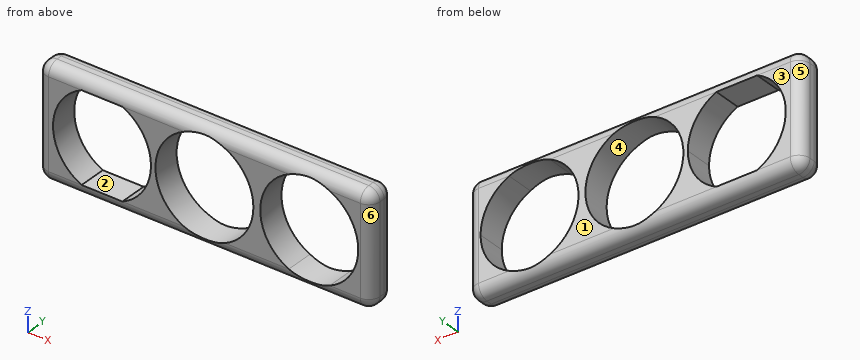
from build123d import *

# Parameters (mm, degrees)
F0_W         = 76.2
F0_H         = 25.4
F0_R         = 11.176
F1_DEPTH     = 6.35
F2_T1_DEPTH  = 71.12
F2_T3_DEPTH  = 1.27
F2_T5_DEPTH  = 20.32
F2_S9_W      = 2.54
F2_S9_H      = 2.54
F2_T10_DEPTH = 2.54
F2_S15_W     = 2.54
F2_S15_H     = 2.54
F2_T16_DEPTH = 2.54
F2_S21_W     = 2.54
F2_S21_H     = 2.54
F2_T22_DEPTH = 2.54
F2_S27_W     = 2.54
F2_S27_H     = 2.54
F2_T28_DEPTH = 2.54
F2_S33_W     = 2.54
F2_S33_H     = 2.54
F2_T34_DEPTH = 2.54
F2_S39_W     = 2.54
F2_S39_H     = 2.54
F2_T40_DEPTH = 2.54
F2_S45_W     = 2.54
F2_S45_H     = 2.54
F2_T46_DEPTH = 2.54
F2_S51_W     = 2.54
F2_S51_H     = 2.54
F2_T52_DEPTH = 2.54
F4_DEPTH     = 6.35


# Not quite as in the source:
# - a fillet or chamfer that OpenCascade refuses, or shapes differently, is made with other operations: its cross-section is extruded or revolved along the edge and cut away or added


with BuildPart() as f1:
    # F0 (on Front) → F1 (new body)
    with BuildSketch(Plane.XZ):
        Rectangle(F0_W, F0_H)
        Circle(F0_R, mode=Mode.SUBTRACT)
    extrude(amount=F1_DEPTH)

    # F2: fillet of radius 2.54 on 12 edges, made by hand

    # F2_s2 → F2_t1 (cut)
    with BuildSketch(Plane.YZ.offset(-35.56)):
        with BuildLine():
            ThreePointArc((-2.54, -12.7), (-0.7439487758, -11.9560512242), (0, -10.16))
            Line((0, -10.16), (0, -12.7))
            Line((0, -12.7), (-2.54, -12.7))
        make_face()
        with BuildLine():
            ThreePointArc((-3.81, -12.7), (-5.6060512242, -11.9560512242), (-6.35, -10.16))
            Line((-6.35, -10.16), (-6.35, -12.7))
            Line((-6.35, -12.7), (-3.81, -12.7))
        make_face()
        with BuildLine():
            ThreePointArc((-2.54, 12.7), (-0.7439487758, 11.9560512242), (0, 10.16))
            Line((0, 10.16), (0, 12.7))
            Line((0, 12.7), (-2.54, 12.7))
        make_face()
        with BuildLine():
            ThreePointArc((-3.81, 12.7), (-5.6060512242, 11.9560512242), (-6.35, 10.16))
            Line((-6.35, 10.16), (-6.35, 12.7))
            Line((-6.35, 12.7), (-3.81, 12.7))
        make_face()
    extrude(amount=F2_T1_DEPTH, mode=Mode.SUBTRACT)

    # F2_s4 → F2_t3 (cut)
    with BuildSketch(Plane.XZ.offset(2.54)):
        with BuildLine():
            ThreePointArc((-38.1, -10.16), (-37.3560512242, -11.9560512242), (-35.56, -12.7))
            Line((-35.56, -12.7), (-38.1, -12.7))
            Line((-38.1, -12.7), (-38.1, -10.16))
        make_face()
        with BuildLine():
            ThreePointArc((38.1, -10.16), (37.3560512242, -11.9560512242), (35.56, -12.7))
            Line((35.56, -12.7), (38.1, -12.7))
            Line((38.1, -12.7), (38.1, -10.16))
        make_face()
        with BuildLine():
            ThreePointArc((38.1, 10.16), (37.3560512242, 11.9560512242), (35.56, 12.7))
            Line((35.56, 12.7), (38.1, 12.7))
            Line((38.1, 12.7), (38.1, 10.16))
        make_face()
        with BuildLine():
            ThreePointArc((-35.56, 12.7), (-37.3560512242, 11.9560512242), (-38.1, 10.16))
            Line((-38.1, 10.16), (-38.1, 12.7))
            Line((-38.1, 12.7), (-35.56, 12.7))
        make_face()
    extrude(amount=F2_T3_DEPTH, mode=Mode.SUBTRACT)

    # F2_s6 → F2_t5 (cut)
    with BuildSketch(Plane.XY.offset(-10.16)):
        with BuildLine():
            ThreePointArc((-38.1, -3.81), (-37.3560512242, -5.6060512242), (-35.56, -6.35))
            Line((-35.56, -6.35), (-38.1, -6.35))
            Line((-38.1, -6.35), (-38.1, -3.81))
        make_face()
        with BuildLine():
            ThreePointArc((-38.1, -2.54), (-37.3560512242, -0.7439487758), (-35.56, 0))
            Line((-35.56, 0), (-38.1, 0))
            Line((-38.1, 0), (-38.1, -2.54))
        make_face()
        with BuildLine():
            ThreePointArc((38.1, -3.81), (37.3560512242, -5.6060512242), (35.56, -6.35))
            Line((35.56, -6.35), (38.1, -6.35))
            Line((38.1, -6.35), (38.1, -3.81))
        make_face()
        with BuildLine():
            ThreePointArc((38.1, -2.54), (37.3560512242, -0.7439487758), (35.56, 0))
            Line((35.56, 0), (38.1, 0))
            Line((38.1, 0), (38.1, -2.54))
        make_face()
    extrude(amount=F2_T5_DEPTH, mode=Mode.SUBTRACT)


with BuildPart() as f2_tool8:
    # F2_s9 → F2_t10 (new body)
    with BuildSketch(Plane.YZ.offset(-35.56)):
        with Locations((-1.27, -11.43)):
            Rectangle(F2_S9_W, F2_S9_H)
    extrude(amount=-F2_T10_DEPTH)

    # F2_s11 → F2_t12 (revolve, cut)
    with BuildSketch(Plane(origin=(-35.56, -2.54, -10.16), x_dir=(0, -0.7071067812, 0.7071067812), z_dir=(0, -0.7071067812, -0.7071067812))):
        with BuildLine():
            ThreePointArc((0, -2.54), (2.54, 0), (0, 2.54))
            Line((0, 2.54), (0, -2.54))
        make_face()
    revolve(axis=Axis((-35.56, -2.54, -10.16), (-1, 0, 0)), mode=Mode.SUBTRACT)


with BuildPart() as f1_1:
    add(f1.part)

    # F2_t7: cut F2_tool8
    add(f2_tool8.part, mode=Mode.SUBTRACT)


with BuildPart() as f2_tool14:
    # F2_s15 → F2_t16 (new body)
    with BuildSketch(Plane.YZ.offset(35.56)):
        with Locations((-1.27, -11.43)):
            Rectangle(F2_S15_W, F2_S15_H)
    extrude(amount=F2_T16_DEPTH)

    # F2_s17 → F2_t18 (revolve, cut)
    with BuildSketch(Plane(origin=(35.56, -2.54, -10.16), x_dir=(0, -0.7071067812, 0.7071067812), z_dir=(0, 0.7071067812, 0.7071067812))):
        with BuildLine():
            ThreePointArc((0, -2.54), (2.54, 0), (0, 2.54))
            Line((0, 2.54), (0, -2.54))
        make_face()
    revolve(axis=Axis((35.56, -2.54, -10.16), (1, 0, 0)), mode=Mode.SUBTRACT)


with BuildPart() as f1_2:
    add(f1_1.part)

    # F2_t13: cut F2_tool14
    add(f2_tool14.part, mode=Mode.SUBTRACT)


with BuildPart() as f2_tool20:
    # F2_s21 → F2_t22 (new body)
    with BuildSketch(Plane.YZ.offset(-35.56)):
        with Locations((-5.08, -11.43)):
            Rectangle(F2_S21_W, F2_S21_H)
    extrude(amount=-F2_T22_DEPTH)

    # F2_s23 → F2_t24 (revolve, cut)
    with BuildSketch(Plane(origin=(-35.56, -3.81, -10.16), x_dir=(0, 0.7071067812, 0.7071067812), z_dir=(0, -0.7071067812, 0.7071067812))):
        with BuildLine():
            ThreePointArc((0, -2.54), (2.54, 0), (0, 2.54))
            Line((0, 2.54), (0, -2.54))
        make_face()
    revolve(axis=Axis((-35.56, -3.81, -10.16), (-1, 0, 0)), mode=Mode.SUBTRACT)


with BuildPart() as f1_3:
    add(f1_2.part)

    # F2_t19: cut F2_tool20
    add(f2_tool20.part, mode=Mode.SUBTRACT)


with BuildPart() as f2_tool26:
    # F2_s27 → F2_t28 (new body)
    with BuildSketch(Plane.YZ.offset(35.56)):
        with Locations((-5.08, -11.43)):
            Rectangle(F2_S27_W, F2_S27_H)
    extrude(amount=F2_T28_DEPTH)

    # F2_s29 → F2_t30 (revolve, cut)
    with BuildSketch(Plane(origin=(35.56, -3.81, -10.16), x_dir=(0, 0.7071067812, 0.7071067812), z_dir=(0, 0.7071067812, -0.7071067812))):
        with BuildLine():
            ThreePointArc((0, -2.54), (2.54, 0), (0, 2.54))
            Line((0, 2.54), (0, -2.54))
        make_face()
    revolve(axis=Axis((35.56, -3.81, -10.16), (1, 0, 0)), mode=Mode.SUBTRACT)


with BuildPart() as f1_4:
    add(f1_3.part)

    # F2_t25: cut F2_tool26
    add(f2_tool26.part, mode=Mode.SUBTRACT)


with BuildPart() as f2_tool32:
    # F2_s33 → F2_t34 (new body)
    with BuildSketch(Plane.XY.offset(10.16)):
        with Locations((-36.83, -5.08)):
            Rectangle(F2_S33_W, F2_S33_H)
    extrude(amount=F2_T34_DEPTH)

    # F2_s35 → F2_t36 (revolve, cut)
    with BuildSketch(Plane(origin=(-35.56, -3.81, 10.16), x_dir=(0.7071067812, 0.7071067812, 0), z_dir=(0.7071067812, -0.7071067812, 0))):
        with BuildLine():
            ThreePointArc((0, -2.54), (2.54, 0), (0, 2.54))
            Line((0, 2.54), (0, -2.54))
        make_face()
    revolve(axis=Axis((-35.56, -3.81, 10.16), (0, 0, 1)), mode=Mode.SUBTRACT)


with BuildPart() as f1_5:
    add(f1_4.part)

    # F2_t31: cut F2_tool32
    add(f2_tool32.part, mode=Mode.SUBTRACT)


with BuildPart() as f2_tool38:
    # F2_s39 → F2_t40 (new body)
    with BuildSketch(Plane.XY.offset(10.16)):
        with Locations((-36.83, -1.27)):
            Rectangle(F2_S39_W, F2_S39_H)
    extrude(amount=F2_T40_DEPTH)

    # F2_s41 → F2_t42 (revolve, cut)
    with BuildSketch(Plane(origin=(-35.56, -2.54, 10.16), x_dir=(0.7071067812, -0.7071067812, 0), z_dir=(-0.7071067812, -0.7071067812, 0))):
        with BuildLine():
            ThreePointArc((0, -2.54), (2.54, 0), (0, 2.54))
            Line((0, 2.54), (0, -2.54))
        make_face()
    revolve(axis=Axis((-35.56, -2.54, 10.16), (0, 0, 1)), mode=Mode.SUBTRACT)


with BuildPart() as f1_6:
    add(f1_5.part)

    # F2_t37: cut F2_tool38
    add(f2_tool38.part, mode=Mode.SUBTRACT)


with BuildPart() as f2_tool44:
    # F2_s45 → F2_t46 (new body)
    with BuildSketch(Plane.YZ.offset(35.56)):
        with Locations((-5.08, 11.43)):
            Rectangle(F2_S45_W, F2_S45_H)
    extrude(amount=F2_T46_DEPTH)

    # F2_s47 → F2_t48 (revolve, cut)
    with BuildSketch(Plane(origin=(35.56, -3.81, 10.16), x_dir=(0, 0.7071067812, -0.7071067812), z_dir=(0, -0.7071067812, -0.7071067812))):
        with BuildLine():
            ThreePointArc((0, -2.54), (2.54, 0), (0, 2.54))
            Line((0, 2.54), (0, -2.54))
        make_face()
    revolve(axis=Axis((35.56, -3.81, 10.16), (1, 0, 0)), mode=Mode.SUBTRACT)


with BuildPart() as f1_7:
    add(f1_6.part)

    # F2_t43: cut F2_tool44
    add(f2_tool44.part, mode=Mode.SUBTRACT)


with BuildPart() as f2_tool50:
    # F2_s51 → F2_t52 (new body)
    with BuildSketch(Plane.YZ.offset(35.56)):
        with Locations((-1.27, 11.43)):
            Rectangle(F2_S51_W, F2_S51_H)
    extrude(amount=F2_T52_DEPTH)

    # F2_s53 → F2_t54 (revolve, cut)
    with BuildSketch(Plane(origin=(35.56, -2.54, 10.16), x_dir=(0, -0.7071067812, -0.7071067812), z_dir=(0, -0.7071067812, 0.7071067812))):
        with BuildLine():
            ThreePointArc((0, -2.54), (2.54, 0), (0, 2.54))
            Line((0, 2.54), (0, -2.54))
        make_face()
    revolve(axis=Axis((35.56, -2.54, 10.16), (1, 0, 0)), mode=Mode.SUBTRACT)


with BuildPart() as f1_8:
    add(f1_7.part)

    # F2_t49: cut F2_tool50
    add(f2_tool50.part, mode=Mode.SUBTRACT)

    # F3 (on face) → F4 (cut)
    with BuildSketch(Plane.XZ.offset(6.35)):
        with BuildLine():
            ThreePointArc((-18.7094612276, -10.16), (-13.9572398788, -6.0369996274), (-12.1859761156, 0))
            ThreePointArc((-12.1859761156, 0), (-13.9572398788, 6.0369996274), (-18.7094612276, 10.16))
            Line((-18.7094612276, 10.16), (-28.0096651758, 10.16))
            ThreePointArc((-28.0096651758, 10.16), (-34.5331502877, 0), (-28.0096651758, -10.16))
            Line((-28.0096651758, -10.16), (-18.7094612276, -10.16))
        make_face()
        with BuildLine():
            ThreePointArc((28.5749689082, -10.16), (33.3248489457, -6.0360861565), (35.0950720022, 0))
            ThreePointArc((35.0950720022, 0), (33.3248489457, 6.0360861565), (28.5749689082, 10.16))
            Line((28.5749689082, 10.16), (19.2631750961, 10.16))
            ThreePointArc((19.2631750961, 10.16), (12.7430720022, 0), (19.2631750961, -10.16))
            Line((19.2631750961, -10.16), (28.5749689082, -10.16))
        make_face()
        with BuildLine():
            Line((19.2631750961, 10.16), (28.5749689082, 10.16))
            ThreePointArc((28.5749689082, 10.16), (23.9190720022, 11.176), (19.2631750961, 10.16))
        make_face()
        with BuildLine():
            ThreePointArc((19.2631750961, -10.16), (23.9190720022, -11.176), (28.5749689082, -10.16))
            Line((28.5749689082, -10.16), (19.2631750961, -10.16))
        make_face()
    extrude(amount=-F4_DEPTH, mode=Mode.SUBTRACT)


solid = f1_8.part
The listing builds one solid part. Answer for the finished solid, in the listing's coordinates (mm). Face numbers are marked on the shaded views. A direction names the side the tool comes from. Give positions to 0.01 mm unless a question says otherwise; leave off trailing zeros. Order: outer loops, then holes, each group sorted by start corner. A loop starts at its lowest first (then second) coordinate and runs counter-clockwise, first axis right, second up. Notation, with made-up numbers: (26.25, 31) -> (42.25, 31) arc R24 cw to (42.25, 63) -> close; hole circle Ø5 at (46.25, 10). An arc over 180 degrees is marked (long way). Put each result on its own line as item: value.
Item 1: A cutting plane is placed at A-A on x = -16.5. Give the vertices of the cut face in (y, z).
Established:
outline: (-6.35, -10.16) arc R2.54 ccw to (-3.81, -12.7) -> (-2.54, -12.7) arc R2.54 ccw to (0, -10.16) -> (0, -8.82) -> (-6.35, -8.82) -> close; (-6.35, 8.82) -> (0, 8.82) -> (0, 10.16) arc R2.54 ccw to (-2.54, 12.7) -> (-3.81, 12.7) arc R2.54 ccw to (-6.35, 10.16) -> close
Item 2: A cutting plane is placed at C-C on y = -5.5. Give the vertices of the cut face in (x, z).
Established:
outline: (-37.46, -10.16) arc R1.9 ccw to (-35.56, -12.06) -> (35.56, -12.06) arc R1.9 ccw to (37.46, -10.16) -> (37.46, 10.16) arc R1.9 ccw to (35.56, 12.06) -> (-35.56, 12.06) arc R1.9 ccw to (-37.46, 10.16) -> close; hole (-28.01, -10.16) -> (-18.71, -10.16) arc R11.17 ccw to (-18.71, 10.16) -> (-28.01, 10.16) arc R11.17 ccw to start; hole circle Ø22.35 at (0, 0); hole circle Ø22.35 at (23.92, 0)
Item 3: A cutting plane is placed at B-B on z = -5.25. Give the vertices of the cut face in (x, y), plus the area to 3 significant figures.
Established:
outline: (-38.1, -3.81) arc R2.54 ccw to (-35.56, -6.35) -> (-33.22, -6.35) -> (-33.22, 0) -> (-35.56, 0) arc R2.54 ccw to (-38.1, -2.54) -> close; (-13.5, -6.35) -> (-9.87, -6.35) -> (-9.87, 0) -> (-13.5, 0) -> close; (9.87, -6.35) -> (14.05, -6.35) -> (14.05, 0) -> (9.87, 0) -> close; (33.79, -6.35) -> (35.56, -6.35) arc R2.54 ccw to (38.1, -3.81) -> (38.1, -2.54) arc R2.54 ccw to (35.56, 0) -> (33.79, 0) -> close
area: 102 mm^2
Item 4: For a pull along X with two mould halves and no side action, classify the marked faces 3, 4, 5 and 6 as released by +X, released by -X, zero draft, split by the parting line, or undercut.
Established:
face 3: zero draft
face 4: undercut
face 5: released by -X
face 6: released by +X
Item 5: Given P1, Ø3, axis at x = 3, y = -5.5, coming from the -Z side, flat-ended and moving along its own axis, determine where the tip first touches the part or whether it passes through.
Established:
P1: stops at z = -12.69
Item 6: A cutting plane is placed at D-D on z = 7.5. Give the vertices of the cut face in (x, y).
Established:
outline: (-38.1, -3.81) arc R2.54 ccw to (-35.56, -6.35) -> (-31.64, -6.35) -> (-31.64, 0) -> (-35.56, 0) arc R2.54 ccw to (-38.1, -2.54) -> close; (-15.08, -6.35) -> (-8.29, -6.35) -> (-8.29, 0) -> (-15.08, 0) -> close; (8.29, -6.35) -> (15.63, -6.35) -> (15.63, 0) -> (8.29, 0) -> close; (32.2, -6.35) -> (35.56, -6.35) arc R2.54 ccw to (38.1, -3.81) -> (38.1, -2.54) arc R2.54 ccw to (35.56, 0) -> (32.2, 0) -> close
Item 7: Straight lines are drawn through the part: line 1 (X direction, y = -4.5, z = -2.25); line 2 (X direction, y = -3.5, z = -9.5); line 3 (Z direction, x = 0, y = -3). For each, find the intervals that lie inside material, in ascending order.
Established:
line 1: x = -38 to -34.3, -12.41 to -10.95, 10.95 to 12.97, 34.87 to 38
line 2: x = -38.1 to -29.24, -17.48 to -5.89, 5.89 to 18.03, 29.81 to 38.1
line 3: z = -12.7 to -11.18, 11.18 to 12.7
Item 8: For the marked faces 1 and 2, determine the directions among +Z, -Z, +X, -X, +Y, -Y from which every point of the face is accessible in a straight line to the end or side of a thin tool.
Established:
face 1: +Z, -Z, +X, -X, +Y
face 2: +Y, -Y
